Part model, mm, in its own coordinate system. Face numbers are marked on the shaded views. A direction names the side the tool comes from. Give positions to 0.01 mm unless a question says otherwise; leave off trailing zeros. Order: outer loops, then holes, each group sorted by start corner. A loop starts at its lowest first (then second) coordinate and runs counter-clockwise, first axis right, second up. Notation, with made-up numbers: M 82.5,-8.75 L 119.5,-8.75 A23 ccw 119.5,-0.75 Z; hole C 57.5,49 d4. An arc over 180 degrees is marked long. Return JSON: item names as keys, results as strings.
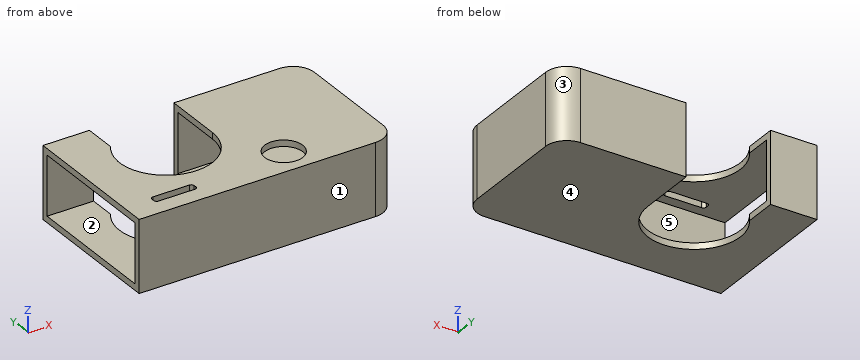
from build123d import *

# Parameters (mm, degrees)
BOSS_EXTRUDE2_DEPTH = 17
CUT_EXTRUDE1_DEPTH  = 14
CUT_EXTRUDE3_DEPTH  = 5
SKETCH9_W           = 14
SKETCH9_H           = 32
CUT_EXTRUDE4_DEPTH  = 11
SKETCH11_R          = 4.5
CUT_EXTRUDE5_DEPTH  = 10.5


with BuildPart() as part:
    # Sketch1 → Boss-Extrude2 (new body)
    with BuildSketch(Plane.XY):
        with BuildLine():
            Line((61, 5), (61, 30))
            ThreePointArc((61, 30), (59.535533906, 33.535533906), (56, 35))
            Line((56, 35), (31, 35))
            Line((31, 35), (31, 21))
            ThreePointArc((31, 21), (16.68337521, 10.511911518), (11, 27.32455532))
            Line((11, 27.32455532), (11, 35))
            Line((11, 35), (0, 35))
            Line((0, 35), (0, 0))
            Line((0, 0), (56, 0))
            ThreePointArc((56, 0), (59.535533906, 1.464466094), (61, 5))
        make_face()
    extrude(amount=BOSS_EXTRUDE2_DEPTH)

    # Sketch5 → Cut-Extrude1 (cut)
    with BuildSketch(Plane(origin=(0, 0, 1.5), x_dir=(-1, 0, 0), z_dir=(0, 0, -1))):
        with BuildLine():
            Line((-54.5, 33.5), (-1.5, 33.5))
            Line((-1.5, 33.5), (-1.5, 1.5))
            Line((-1.5, 1.5), (-54.5, 1.5))
            ThreePointArc((-54.5, 1.5), (-58.035533906, 2.964466094), (-59.5, 6.5))
            Line((-59.5, 6.5), (-59.5, 28.5))
            ThreePointArc((-59.5, 28.5), (-58.035533906, 32.035533906), (-54.5, 33.5))
        make_face()
    extrude(amount=-CUT_EXTRUDE1_DEPTH, mode=Mode.SUBTRACT)

    # Sketch10 → Cut-Extrude3 (cut)
    with BuildSketch(Plane.XY.offset(17)):
        with BuildLine():
            Line((7.2, 4), (15.8, 4))
            ThreePointArc((15.8, 4), (16.294974747, 4.205025253), (16.5, 4.7))
            Line((16.5, 4.7), (16.5, 5.3))
            ThreePointArc((16.5, 5.3), (16.294974747, 5.794974747), (15.8, 6))
            Line((15.8, 6), (7.2, 6))
            ThreePointArc((7.2, 6), (6.705025253, 5.794974747), (6.5, 5.3))
            Line((6.5, 5.3), (6.5, 4.7))
            ThreePointArc((6.5, 4.7), (6.705025253, 4.205025253), (7.2, 4))
        make_face()
    extrude(amount=-CUT_EXTRUDE3_DEPTH, mode=Mode.SUBTRACT)

    # Sketch9 → Cut-Extrude4 (cut)
    with BuildSketch(Plane.ZY):
        with Locations((8.5, 17.5)):
            Rectangle(SKETCH9_W, SKETCH9_H)
    extrude(amount=-CUT_EXTRUDE4_DEPTH, mode=Mode.SUBTRACT)

    # Sketch11 → Cut-Extrude5 (cut)
    with BuildSketch(Plane.XY.offset(17)):
        with Locations((38.8, 7)):
            Circle(SKETCH11_R)
    extrude(amount=-CUT_EXTRUDE5_DEPTH, mode=Mode.SUBTRACT)


solid = part.part
Q1. Two-plate mould, pull along Z, no slides. Class the marked faces 3, 4 and 5: +Z half, -Z half, draft (parallel to the pull), parting line (faces both ways), or undercut.
Established:
{"face 3": "draft", "face 4": "-Z half", "face 5": "undercut"}
Q2. Band-saw the part on C-C (y = 22). Give the cut face in (x, z).
Established:
{"outline": "M 0,0 L 9.05,0 L 9.05,1.5 L 0,1.5 Z; M 0,15.5 L 9.05,15.5 L 9.05,17 L 0,17 Z; M 31,0 L 61,0 L 61,17 L 31,17 L 31,15.5 L 59.5,15.5 L 59.5,1.5 L 31,1.5 Z"}
Q3. 3-axis set-ups, long thin cutter, end or side, ignore diameter. For the marked faces 1 and 2: which of +Z, -Z, +X, -X, +Y, -Y reach the whole face in a straight line?
Established:
{"face 1": "+Z, -Z, +X, -X, -Y", "face 2": "-X"}
Q4. Pin check, flat tips, straight feed: pin 1 (2.5 mm diameter, centred on y = 32, z = 10.5, fed in from +X); pin 2 (4 mm diameter, centred on y = 15.5, z = 12, fed in from -X). Stop position of each tip, or through.
Established:
{"pin 1": "stops at x = 60.94", "pin 2": "stops at x = 59.5"}
Q5. Probe line 1 along Y through (x, z) = (47, 7.5); line 2 along Z through (x, y) = (16.5, 7); line 3 along Y through (x, z) = (28, 10.75). List the from-to ranges inside material, lowest first.
Established:
{"line 1": "y = 0 to 1.5, 33.5 to 35", "line 2": "z = 0 to 1.5, 15.5 to 17", "line 3": "y = 0 to 1.5"}
Q6. Band-saw the part on B-B (z = 12). Give the cut face in (x, y), then the cut area to 3 significant figures.
Established:
{"outline": "M 0,0 L 56,0 A5 ccw 61,5 L 61,30 A5 ccw 56,35 L 31,35 L 31,33.5 L 54.5,33.5 A5 cw 59.5,28.5 L 59.5,6.5 A5 cw 54.5,1.5 L 0,1.5 Z; M 0,33.5 L 11,33.5 L 11,35 L 0,35 Z", "area": "201 mm²"}
Q7. Band-saw the part on D-D (x = 20). Give the cut face in (y, z).
Established:
{"outline": "M 0,0 L 10,0 L 10,1.5 L 1.5,1.5 L 1.5,15.5 L 10,15.5 L 10,17 L 0,17 Z"}
Q8. Band-saw the part on A-A (x = 50). Give the cut face in (y, z).
Established:
{"outline": "M 0,0 L 35,0 L 35,17 L 0,17 Z; hole M 1.5,1.5 L 33.5,1.5 L 33.5,15.5 L 1.5,15.5 Z"}
